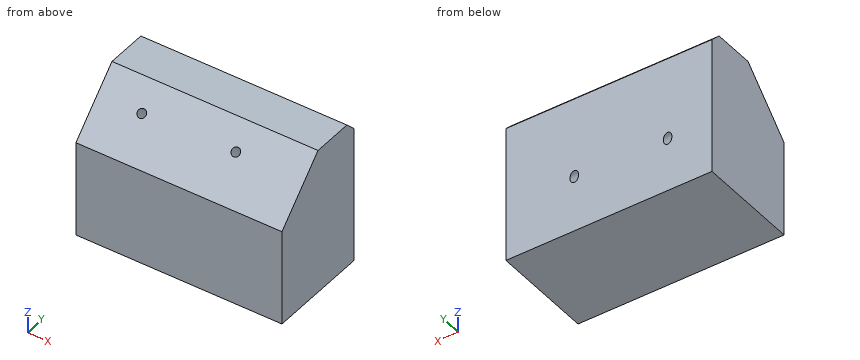
from build123d import *

# Parameters (mm, degrees)
F0_W     = 100
F0_H     = 50
F1_DEPTH = 71.6
F2_SIZE  = 25
F4_D     = 4.2
F5_SIZE  = 5


with BuildPart() as f1:
    # F0 (on Top) → F1 (new body)
    with BuildSketch(Plane.XY):
        with Locations((50, 25)):
            Rectangle(F0_W, F0_H)
    extrude(amount=F1_DEPTH)

    # F2
    f2_edges = [f1.edges().sort_by_distance(p)[0] for p in [
        (50, 0, 71.6),
    ]]
    chamfer(f2_edges, length=F2_SIZE)

    # F4 (through all)
    with Locations(Plane(origin=(0, -23.3, 23.3), x_dir=(1, 0, 0), z_dir=(0, -0.7071067812, 0.7071067812))):
        with Locations((66.7982175946, 54.7630861402), (21.5294957161, 54.0269054472)):
            Hole(F4_D / 2)

    # F5
    f5_edges = [f1.edges().sort_by_distance(p)[0] for p in [
        (50, 50, 71.6),
    ]]
    chamfer(f5_edges, length=F5_SIZE)


solid = f1.part
Can you work these out from the model? Positions are in its coordinate system, mm. Give positions to 0.01 mm unless a question says otherwise; leave off trailing zeros. Loops run counter-clockwise (first coordinate to the right, second up) from the corner with the lowest first, then second, coordinate; pieces in that order, holes last. Notation, with made-up numbers: (66.25, 88) - (74.25, 88) arc R21 cw to (74.25, 124) - close; hole circle Ø6 at (23.5, 21). An arc over 180 degrees is marked (long way). Return JSON: item names as keys, results as strings.
1. I want a section at C-C on y = 10. Please give me the cut outline in (x, z), and give its area (3 significant figures).
Output values:
{"outline": "(0, 0) - (100, 0) - (100, 56.6) - (0, 56.6) - close", "area": "5,660 mm²"}
2. If I drill on line 1 (Z direction, x = 87.5, y = 5); line 2 (Z direction, x = 13, y = 24); line 3 (Y direction, x = 8.5, z = 59), over which ranges is the centre line in solid material (lowest first)?
Output values:
{"line 1": "z = 0 to 51.6", "line 2": "z = 0 to 70.6", "line 3": "y = 12.4 to 50"}
3. I want a section at D-D on z = 59. Give the number of separate pieces and of enclosed holes in the cut face, and give its area (3 significant figures).
Output values:
{"separate pieces": "1", "enclosed holes": "2", "area": "3,720 mm²"}
4. I want a section at A-A on x = 67. Please give me the cut outline in (y, z).
Output values:
{"outline": "(0, 0) - (50, 0) - (50, 24.49) - (13.95, 60.55) - (0, 46.6) - close; (16.9, 63.5) - (50, 30.4) - (50, 66.6) - (45, 71.6) - (25, 71.6) - close"}
5. I want a section at B-B on x = 36. Please give me the cut outline in (y, z).
Output values:
{"outline": "(0, 0) - (50, 0) - (50, 66.6) - (45, 71.6) - (25, 71.6) - (0, 46.6) - close"}
6. I'm going to push flat-ended pins straight in: pin 1 Ø1 at (x, y) = (49, 13) entering from +Z; pin 2 Ø12 at (x, z) = (49.5, 54.5) entering from -Y. Where does each tip first touch, or does it pass through?
Output values:
{"pin 1": "stops at z = 60.1", "pin 2": "stops at y = 1.9"}
